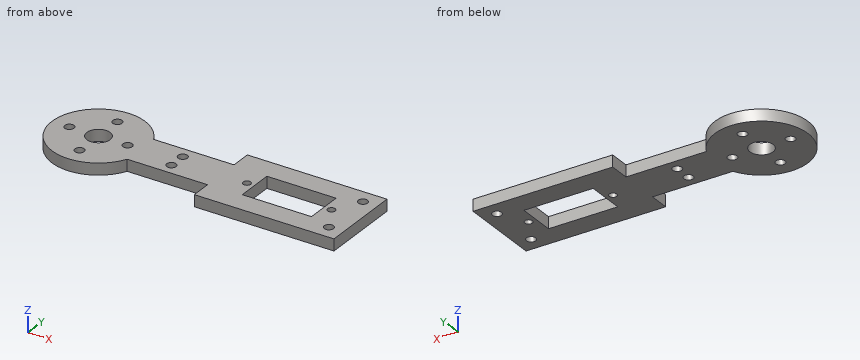
```python
from build123d import *

# Parameters (mm, degrees)
MAIN_WEB_PROFILE_W                     = 60
MAIN_WEB_PROFILE_H                     = 14
MAIN_WEB_DEPTH                         = 4
SHOULDER_HORN_FLANGE_PROFILE_R         = 16
SHOULDER_HORN_FLANGE_DEPTH             = 4
ELBOW_SERVO_MOUNT_PROFILE_W            = 48
ELBOW_SERVO_MOUNT_PROFILE_H            = 28
ELBOW_SERVO_MOUNT_DEPTH                = 4
SG90_BODY_CLEARANCE_START              = -5
SG90_BODY_CLEARANCE_PROFILE_W          = 23.8
SG90_BODY_CLEARANCE_PROFILE_H          = 13
SG90_BODY_CLEARANCE_DEPTH              = 97.49863387
ELBOW_TAB_FASTENERS_START              = -50
ELBOW_TAB_FASTENERS_PROFILE_R          = 1.3
ELBOW_TAB_FASTENERS_DEPTH              = 142.49863387
SHOULDER_CENTER_SCREW_ACCESS_START     = -50
SHOULDER_CENTER_SCREW_ACCESS_PROFILE_R = 4
SHOULDER_CENTER_SCREW_ACCESS_DEPTH     = 142.49863387
SHOULDER_HORN_BOLT_PATTERN_START       = -50
SHOULDER_HORN_BOLT_PATTERN_PROFILE_R   = 1.6
SHOULDER_HORN_BOLT_PATTERN_DEPTH       = 142.49863387
CABLE_TIE_HOLES_START                  = -50
CABLE_TIE_HOLES_PROFILE_R              = 1.6
CABLE_TIE_HOLES_DEPTH                  = 142.49863387
PASSIVE_CHEEK_STANDOFFS_START          = -50
PASSIVE_CHEEK_STANDOFFS_PROFILE_R      = 1.6
PASSIVE_CHEEK_STANDOFFS_DEPTH          = 142.49863387


with BuildPart() as part:
    # Main_web_profile → Main_web (new body)
    with BuildSketch(Plane.XY):
        with Locations((30, 0)):
            Rectangle(MAIN_WEB_PROFILE_W, MAIN_WEB_PROFILE_H)
    extrude(amount=MAIN_WEB_DEPTH)

    # Shoulder_horn_flange_profile → Shoulder_horn_flange (add)
    with BuildSketch(Plane.XY):
        Circle(SHOULDER_HORN_FLANGE_PROFILE_R)
    extrude(amount=SHOULDER_HORN_FLANGE_DEPTH)

    # Elbow_servo_mount_profile → Elbow_servo_mount (add)
    with BuildSketch(Plane.XY):
        with Locations((66, 0)):
            Rectangle(ELBOW_SERVO_MOUNT_PROFILE_W, ELBOW_SERVO_MOUNT_PROFILE_H)
    extrude(amount=ELBOW_SERVO_MOUNT_DEPTH)

    # SG90_body_clearance_profile → SG90_body_clearance (cut, through all)
    with BuildSketch(Plane.XY.offset(SG90_BODY_CLEARANCE_START)):
        with Locations((65.5, 0)):
            Rectangle(SG90_BODY_CLEARANCE_PROFILE_W, SG90_BODY_CLEARANCE_PROFILE_H)
    extrude(amount=SG90_BODY_CLEARANCE_DEPTH, mode=Mode.SUBTRACT)

    # Elbow_tab_fasteners_profile → Elbow_tab_fasteners (cut, through all)
    with BuildSketch(Plane.XY.offset(ELBOW_TAB_FASTENERS_START)):
        with Locations(Location((51, 0, 0), (0, 0, 180))):
            Circle(ELBOW_TAB_FASTENERS_PROFILE_R)
        with Locations(Location((80, 0, 0), (0, 0, 180))):
            Circle(ELBOW_TAB_FASTENERS_PROFILE_R)
    extrude(amount=ELBOW_TAB_FASTENERS_DEPTH, mode=Mode.SUBTRACT)

    # Shoulder_center_screw_access_profile → Shoulder_center_screw_access (cut, through all)
    with BuildSketch(Plane.XY.offset(SHOULDER_CENTER_SCREW_ACCESS_START)):
        with Locations(Location((0, 0, 0), (0, 0, 180))):
            Circle(SHOULDER_CENTER_SCREW_ACCESS_PROFILE_R)
    extrude(amount=SHOULDER_CENTER_SCREW_ACCESS_DEPTH, mode=Mode.SUBTRACT)

    # Shoulder_horn_bolt_pattern_profile → Shoulder_horn_bolt_pattern (cut, through all)
    with BuildSketch(Plane.XY.offset(SHOULDER_HORN_BOLT_PATTERN_START)):
        with Locations(Location((0, 10, 0), (0, 0, 180))):
            Circle(SHOULDER_HORN_BOLT_PATTERN_PROFILE_R)
        with Locations(Location((0, -10, 0), (0, 0, 180))):
            Circle(SHOULDER_HORN_BOLT_PATTERN_PROFILE_R)
        with Locations(Location((10, 0, 0), (0, 0, 180))):
            Circle(SHOULDER_HORN_BOLT_PATTERN_PROFILE_R)
        with Locations(Location((-10, 0, 0), (0, 0, 180))):
            Circle(SHOULDER_HORN_BOLT_PATTERN_PROFILE_R)
    extrude(amount=SHOULDER_HORN_BOLT_PATTERN_DEPTH, mode=Mode.SUBTRACT)

    # Cable_tie_holes_profile → Cable_tie_holes (cut, through all)
    with BuildSketch(Plane.XY.offset(CABLE_TIE_HOLES_START)):
        with Locations(Location((27, -3, 0), (0, 0, 180))):
            Circle(CABLE_TIE_HOLES_PROFILE_R)
        with Locations(Location((27, 3, 0), (0, 0, 180))):
            Circle(CABLE_TIE_HOLES_PROFILE_R)
    extrude(amount=CABLE_TIE_HOLES_DEPTH, mode=Mode.SUBTRACT)

    # Passive_cheek_standoffs_profile → Passive_cheek_standoffs (cut, through all)
    with BuildSketch(Plane.XY.offset(PASSIVE_CHEEK_STANDOFFS_START)):
        with Locations(Location((85, -9, 0), (0, 0, 180))):
            Circle(PASSIVE_CHEEK_STANDOFFS_PROFILE_R)
        with Locations(Location((85, 9, 0), (0, 0, 180))):
            Circle(PASSIVE_CHEEK_STANDOFFS_PROFILE_R)
    extrude(amount=PASSIVE_CHEEK_STANDOFFS_DEPTH, mode=Mode.SUBTRACT)


solid = part.part
```
Verification items for the finished model (mm, model axes). Coordinates: 2 decimals unless noted, no trailing zeros. Write each loop counter-clockwise with the first axis right and the second up, starting at its lowest first coordinate (ties: lowest second). Pieces come first, ordered by that corner, then holes. Notation, with made-up numbers: (9, 21.5) - (67, 21.5) arc R8 cw to (67, 36.5) - close; hole circle Ø6 at (88, 15.25). An arc over 180 degrees is marked (long way). Write item = value, one per line.
Q1. Go/stop test with flat-tipped pins: pin 1 Ø1.5 at (x, z) = (70.5, 3.5) entering from +Y; pin 2 Ø2 at (x, z) = (28.5, 3) entering from -Y; pin 3 Ø1.6 at (x, y) = (80, 0) entering from +Z; pin 4 Ø1.2 at (x, z) = (56.5, 3) entering from -Y. Record where each tip stops, or that it passes through.
Answer:
pin_1 = 14
pin_2 = -7
pin_3 = through
pin_4 = -14
Q2. Material ranges on L1, parallel to Y at x = 0, z = 1.75; L2, parallel to Y at x = 71.5, z = 0.6; L3, parallel to Y at x = 51, z = 2.25, recorded low to high. Write a range as from..to.
Answer:
L1 = -16..-11.6, -8.4..-4, 4..8.4, 11.6..16
L2 = -14..-6.5, 6.5..14
L3 = -14..-1.3, 1.3..14
Q3. Cross-section at A-A (x = 0). Enter the section's corners in (y, z), plus the area to 3 significant figures.
Answer:
outline = (-16, 0) - (-11.6, 0) - (-11.6, 4) - (-16, 4) - close; (-8.4, 0) - (-4, 0) - (-4, 4) - (-8.4, 4) - close; (4, 0) - (8.4, 0) - (8.4, 4) - (4, 4) - close; (11.6, 0) - (16, 0) - (16, 4) - (11.6, 4) - close
area = 70.4 mm²
Q4. Cross-section at B-B (x = 51). Enter the section's corners in (y, z), plus the area to 3 significant figures.
Answer:
outline = (-14, 0) - (-1.3, 0) - (-1.3, 4) - (-14, 4) - close; (1.3, 0) - (14, 0) - (14, 4) - (1.3, 4) - close
area = 102 mm²
Q5. Cross-section at C-C (y = 0). Enter the section's corners in (x, z), plus the area to 3 significant figures.
Answer:
outline = (-16, 0) - (-11.6, 0) - (-11.6, 4) - (-16, 4) - close; (-8.4, 0) - (-4, 0) - (-4, 4) - (-8.4, 4) - close; (4, 0) - (8.4, 0) - (8.4, 4) - (4, 4) - close; (11.6, 0) - (49.7, 0) - (49.7, 4) - (11.6, 4) - close; (52.3, 0) - (53.6, 0) - (53.6, 4) - (52.3, 4) - close; (77.4, 0) - (78.7, 0) - (78.7, 4) - (77.4, 4) - close; (81.3, 0) - (90, 0) - (90, 4) - (81.3, 4) - close
area = 250 mm²
Q6. Cross-section at D-D (z = 1). Give the number of separate pieces and of enclosed holes in the cut face, plus the area to 3 significant figures.
Answer:
separate_pieces = 1
enclosed_holes = 12
area = 2,080 mm²
